from build123d import *

# Parameters (mm, degrees)
F1_DEPTH = 19.05
F3_D     = 6.35
F4_R     = 6.35


with BuildPart() as f1:
    # F0 (on Front) → F1 (new body)
    with BuildSketch(Plane.XZ):
        Polygon((-19.05, 0), (0, 0), (12.7, 0), (12.7, 27.648715), (0, 27.648715), (0, 12.7), (-19.05, 12.7), align=None)
    extrude(amount=F1_DEPTH)

    # F3 (through all)
    with Locations(Plane.XY.offset(12.7)):
        with Locations((-9.525, -9.525)):
            Hole(F3_D / 2)

    # F4
    f4_edges = [f1.edges().sort_by_distance(p)[0] for p in [
        (-19.05, 0, 6.35),
        (-19.05, -19.05, 6.35),
    ]]
    fillet(f4_edges, radius=F4_R)

    # F5: F1 across face


with BuildPart() as f1_1:
    add(f1.part)
    add(f1.part.mirror(Plane(origin=(12.7, -9.525, 13.824358), x_dir=(0, 1, 0), z_dir=(1, 0, 0))))


solid = f1_1.part
Source: CAD feature listing. Evaluate the final solid. Frame: model axes, mm. A direction names the side the tool comes from. Round coordinates to 2 decimals unless told otherwise and drop trailing zeros. Loops run counter-clockwise (first coordinate to the right, second up) from the corner with the lowest first, then second, coordinate; pieces in that order, holes last. Notation, with made-up numbers: M -28,65 L -2,65 A25 cw -2,85 Z; hole C -24.5,11 d4. An arc over 180 degrees is marked long. Return JSON: item names as keys, results as strings. Group by question number.
1. Pin query (flat end, axial travel): pin 1 (7.5 mm diameter, centred on y = -11, z = 20, fed in from -X); pin 2 (1.5 mm diameter, centred on y = -17, z = 4.5, fed in from -X) (3 decimals); pin 3 (1 mm diameter, centred on y = -15.5, z = 8, fed in from +X); pin 4 (4 mm diameter, centred on x = 34.925, y = -9.525, fed in from -Z). Return the tip coordinate at first contact, or that it passes through.
2. Section query D-D on x = -11. Output: boundary loops of the cut face in (y, z).
3. Section query C-C on z = 2.5. Output: boundary loops of the cut face in (x, y) (3 decimals).
4. Section query B-B on y = -14. Output: boundary loops of the cut face in (x, z), and give its area (3 significant figures).
5. Material intervals for line 1 along Z through (x, y) = (38, -5.75); line 2 along X through (y, z) = (-7, 18.25); line 3 along X through (y, z) = (-14.5, 6.75), sorted ascending. Write a range as from..to.
6. Mould query, pull axis X, two halves, no side actions, for faces 1 (the face through (13, 0, 11)), 2 (the face through (42.64, -1.91, 6.26)), 3 (the face through (-12.46, -10.74, 6.26)). Classes: released by +X, released by -X, zero draft, split by the parting line, or undercut.
7. Reachability of faces 4 (the face through (25.4, -9, 20)), 5 (the face through (13, -9, 27.649)), 6 (the face through (0, -9, 20)) from +Z, -Z, +X, -X, +Y, -Y: full face, straight path, thin tool, end or side. Return the list, or none.
8. Section query A-A on x = 33.5. Output: boundary loops of the cut face in (y, z).
Checks:
{
 "1": {"pin 1": "stops at x = 0", "pin 2": "stops at x = -17.965", "pin 3": "stops at x = 44.02", "pin 4": "passes through"},
 "2": {"outline": "M -19.05,0 L -12.34,0 L -12.34,12.7 L -19.05,12.7 Z; M -6.71,0 L 0,0 L 0,12.7 L -6.71,12.7 Z"},
 "3": {"outline": "M -19.05,-12.7 A6.35 ccw -12.7,-19.05 L 38.1,-19.05 A6.35 ccw 44.45,-12.7 L 44.45,-6.35 A6.35 ccw 38.1,0 L -12.7,0 A6.35 ccw -19.05,-6.35 Z; hole C -9.525,-9.525 d6.35; hole C 34.925,-9.525 d6.35"},
 "4": {"outline": "M -18.92,0 L 44.32,0 L 44.32,12.7 L 25.4,12.7 L 25.4,27.65 L 0,27.65 L 0,12.7 L -18.92,12.7 Z", "area": "1,180 mm²"},
 "5": {"line 1": "z = 0..12.7", "line 2": "x = 0..25.4", "line 3": "x = -18.79..44.19"},
 "6": {"face 1": "zero draft", "face 2": "released by +X", "face 3": "undercut"},
 "7": {"face 4": "+Z, +X, +Y, -Y", "face 5": "+Z, +X, -X, +Y, -Y", "face 6": "+Z, -X, +Y, -Y"},
 "8": {"outline": "M -19.05,0 L -12.36,0 L -12.36,12.7 L -19.05,12.7 Z; M -6.69,0 L 0,0 L 0,12.7 L -6.69,12.7 Z"}
}
